```python
from build123d import *

# Parameters (mm, degrees)
SKETCH_1_R          = 25
EXTRUDE_1_DEPTH     = 12
SKETCH_2_R          = 13
EXTRUDE_2_DEPTH     = 13
SKETCH_3_R          = 4
CUT_EXTRUDE_1_DEPTH = 13


with BuildPart() as part:
    # 草图1 → 凸台-拉伸1 (new body)
    with BuildSketch(Plane.XY):
        Circle(SKETCH_1_R)
    extrude(amount=EXTRUDE_1_DEPTH)

    # 草图2 → 凸台-拉伸2 (add)
    with BuildSketch(Plane(origin=(0, 0, 0), x_dir=(-1, 0, 0), z_dir=(0, 0, -1))):
        Circle(SKETCH_2_R)
    extrude(amount=EXTRUDE_2_DEPTH)

    # 草图3 → 切除-拉伸1 (cut)
    with BuildSketch(Plane(origin=(0, 0, -13), x_dir=(-1, 0, 0), z_dir=(0, 0, -1))):
        Circle(SKETCH_3_R)
    extrude(amount=-CUT_EXTRUDE_1_DEPTH, mode=Mode.SUBTRACT)

    # 草图4 → 旋转1 (revolve)
    with BuildSketch(Plane(origin=(0, 0, 0), x_dir=(0, 0, -1), z_dir=(1, 0, 0))):
        Polygon((-12, 22.5), (-21, 24), (-31, 24), (-31, 20), (-12, 20), align=None)
    revolve(axis=Axis((0, 20, 31), (0, 0, -1)))


solid = part.part
```
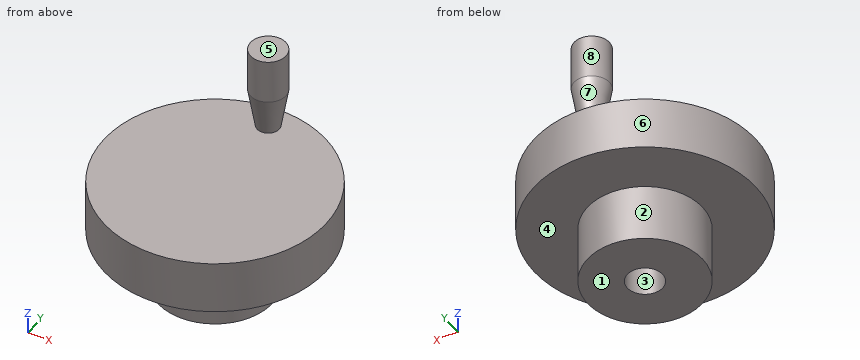
The model under review builds one solid part; all positions refer to its coordinate system, in mm. Face numbers are marked on the shaded views. A direction names the side the tool comes from. Give positions to 0.01 mm unless a question says otherwise; leave off trailing zeros. Write each loop counter-clockwise with the first axis right and the second up, starting at its lowest first coordinate (ties: lowest second). Pieces come first, ordered by that corner, then holes. Notation, with made-up numbers: (-32.75, 71.5) - (10.25, 71.5) arc R25 ccw to (10.25, 94.5) - close; hole circle Ø4 at (-24.75, 18.5). An arc over 180 degrees is marked (long way). Answer in a Markdown table with one row per item. Add a question column.
1. We need section A-A on y = 0. Write out the cut boundary in (x, z).
2. We need section C-C on z = -5. Write out the cut boundary in (x, y).
3. We need section B-B on x = 0. Write out the cut boundary in (y, z), then the cut area to 4 significant figures.
4. We need section D-D on z = 10.5. Write out the cut boundary in (x, y), then the cut area to 3 significant figures.
5. Draft analysis for pull direction X (two halves, no side actions). For the marked faces 1, 2 and 3, state which applies: +X half, -X half, draft (parallel to the pull), parting line (faces both ways), or undercut.
6. Insertion check: P1, Ø15, axis at x = -6, y = -4.5, coming from the +Z side; P2, Ø10, axis at x = 18.5, y = -19.5, coming from the -Z side; P3, Ø8, axis at y = 17, z = 11.5, coming from the -X side. Each pin has a flat end and moves straight along its axis. Give the tip position at first contact, or say it passes through.
7. Tool access review of the marked faces 4, 5, 6, 7 and 8: name each direction out of +Z, -Z, +X, -X, +Y, -Y from which nothing blocks a thin tool from reaching the whole face with its end or side.
8. Wall thickness on line 1 along Y through (x, z) = (0, -5.75); line 2 along Z through (x, y) = (21, -11); line 3 along Z through (x, y) = (-11, -0.5): over which ranges is each line inside the solid? List them lowest first. Write a range as [from, to].
Ans:
| question | item | result |
|---|---|---|
| 1 | outline | (-25, 0) - (-13, 0) - (-13, -13) - (-4, -13) - (-4, 0) - (4, 0) - (4, -13) - (13, -13) - (13, 0) - (25, 0) - (25, 12) - (-25, 12) - close |
| 2 | outline | circle Ø26 at (0, 0); hole circle Ø8 at (0, 0) |
| 3 | outline | (-25, 0) - (-13, 0) - (-13, -13) - (-4, -13) - (-4, 0) - (4, 0) - (4, -13) - (13, -13) - (13, 0) - (25, 0) - (25, 12) - (22.5, 12) - (24, 21) - (24, 31) - (16, 31) - (16, 21) - (17.5, 12) - (-25, 12) - close |
| 3 | area | 972.5 mm^2 |
| 4 | outline | circle Ø50 at (0, 0) |
| 4 | area | 1,960 mm^2 |
| 5 | face 1 | draft |
| 5 | face 2 | parting line |
| 5 | face 3 | undercut |
| 6 | P1 | stops at z = 12 |
| 6 | P2 | stops at z = 0 |
| 6 | P3 | stops at x = -21.35 |
| 7 | face 4 | -Z |
| 7 | face 5 | +Z, +X, -X, +Y, -Y |
| 7 | face 6 | +Z, -Z |
| 7 | face 7 | none |
| 7 | face 8 | +Z |
| 8 | line 1 | y = [-13, -4], [4, 13] |
| 8 | line 2 | z = [0, 12] |
| 8 | line 3 | z = [-13, 12] |
